Could you check a few things on this model? Use its own coordinates, in mm. Face numbers are marked on the shaded views. A direction names the side the tool comes from. Round coordinates to 2 decimals unless told otherwise and drop trailing zeros. Loops run counter-clockwise (first coordinate to the right, second up) from the corner with the lowest first, then second, coordinate; pieces in that order, holes last. Notation, with made-up numbers: (71.25, 72.5) -> (111.25, 72.5) arc R16 ccw to (111.25, 96.5) -> close; hole circle Ø1 at (51.5, 27). An arc over 180 degrees is marked (long way). Put each result on its own line as item: value. Start each with the question number.
1. I'm going to push flat-ended pins straight in: P1, Ø5, axis at x = -14, y = -21, coming from the +Z side; P2, Ø5, axis at x = 13, y = 12, coming from the -Z side; P3, Ø6, axis at x = 2, z = -4, coming from the -Y side. Where does each tip first touch, or does it pass through?
2. If we mould it in two halves opening along Z, with no side actions, what happens to the marked faces 4, 5 and 6? For each: pulls with the +Z half, pulls with the -Z half, needs draft (parallel to the pull), parting line crosses it, or undercut.
3. Which directions (+Z, -Z, +X, -X, +Y, -Y) give clear straight access to the entire face, cutting with the end or side of a thin tool? Please do the marked faces 1, 2 and 3.
4. Imagine slicing it at A-A, the plane y = 24.75. Please give me the cut outline in (x, z).
5. Imagine slicing it at B-B, the plane x = -24.75. Please give me the cut outline in (y, z).
6. Imagine slicing it at C-C, the plane z = 11. Please give me the cut outline in (x, y).
7. Imagine slicing it at D-D, the plane x = 0. Please give me the cut outline in (y, z).
8. I need wall thicknesses on line 1 (Y direction, x = -24.75, z = 28.5); line 2 (Z direction, x = -0.5, y = 3.5); line 3 (Y direction, x = -24, z = 8). Which ranges of each line are inside material? Lowest first, please. Write a range as [from, to].
```python
from build123d import *

# Parameters (mm, degrees)
BOSS_EXTRUDE1_DEPTH = 2.5
SKETCH3_W           = 45
SKETCH3_H           = 1.418134712
SKETCH3_W_2         = 44.463900584
SKETCH3_H_2         = 3.684459624
BOSS_EXTRUDE2_DEPTH = 31.5
SKETCH4_W           = 60.536099416
SKETCH4_H           = 60
BOSS_EXTRUDE3_DEPTH = 34
SKETCH5_R           = 21
BOSS_EXTRUDE4_DEPTH = 80
SKETCH6_R           = 4
BOSS_EXTRUDE5_DEPTH = 3
SKETCH7_R           = 15
BOSS_EXTRUDE6_DEPTH = 22
SKETCH13_R          = 2
CUT_EXTRUDE1_DEPTH  = 3
CUT_EXTRUDE2_START  = -3
SKETCH14_R          = 2
CUT_EXTRUDE2_DEPTH  = 3
SKETCH15_R          = 2.5
SKETCH15_W          = 52.231950292
SKETCH15_H          = 11.081865288
SKETCH15_W_2        = 52.768049708
SKETCH15_H_2        = 8.918134712
CUT_EXTRUDE3_DEPTH  = 128.185394164


with BuildPart() as part:
    # Sketch2 → Boss-Extrude1 (new body)
    with BuildSketch(Plane.XY):
        Polygon((-30.268049708, -30), (-30.268049708, 31.081865288), (-22.5, 31.081865288), (-22.5, 41.081865288), (21.963900584, 41.081865288), (21.963900584, 29.468648207), (29.731950292, 29.468648207), (29.731950292, -30.531351793), (22.5, -30.531351793), (22.5, -38.918134712), (-22.5, -38.918134712), (-22.5, -30), align=None)
    extrude(amount=BOSS_EXTRUDE1_DEPTH)

    # Sketch3 → Boss-Extrude2 (add)
    with BuildSketch(Plane.XY.offset(2.5)):
        with Locations((0, -38.209067356)):
            Rectangle(SKETCH3_W, SKETCH3_H)
        with Locations((-0.268049708, 39.239635476)):
            Rectangle(SKETCH3_W_2, SKETCH3_H_2)
    extrude(amount=BOSS_EXTRUDE2_DEPTH)

    # Sketch4 → Boss-Extrude3 (add)
    with BuildSketch(Plane.XY.offset(2.5)):
        Rectangle(SKETCH4_W, SKETCH4_H)
    extrude(amount=BOSS_EXTRUDE3_DEPTH)

    # Sketch5 → Boss-Extrude4 (add)
    with BuildSketch(Plane.XY.offset(36.5)):
        Circle(SKETCH5_R)
    extrude(amount=BOSS_EXTRUDE4_DEPTH)

    # Sketch6 → Boss-Extrude5 (add)
    with BuildSketch(Plane(origin=(0, 0, 0), x_dir=(-1, 0, 0), z_dir=(0, 0, -1))):
        with Locations((0, -10)):
            Circle(SKETCH6_R)
    extrude(amount=BOSS_EXTRUDE5_DEPTH)

    # Sketch7 → Boss-Extrude6 (add)
    with BuildSketch(Plane(origin=(0, 0, -3), x_dir=(-1, 0, 0), z_dir=(0, 0, -1))):
        with Locations((0, -10)):
            Circle(SKETCH7_R)
    extrude(amount=BOSS_EXTRUDE6_DEPTH)

    # Sketch13 → Cut-Extrude1 (cut)
    with BuildSketch(Plane(origin=(0, 41.081865288, 0), x_dir=(1, 0, 0), z_dir=(0, 1, 0))):
        with Locations(Location((-12.5, -14, 0), (0, 0, 270))):
            Circle(SKETCH13_R)
        with Locations(Location((12.5, -14, 0), (0, 0, 270))):
            Circle(SKETCH13_R)
        with Locations(Location((-12.5, -26, 0), (0, 0, 270))):
            Circle(SKETCH13_R)
        with Locations(Location((12.5, -26, 0), (0, 0, 270))):
            Circle(SKETCH13_R)
    extrude(amount=-CUT_EXTRUDE1_DEPTH, mode=Mode.SUBTRACT)

    # Sketch14 → Cut-Extrude2 (cut)
    with BuildSketch(Plane.XZ.offset(38.918134712).offset(CUT_EXTRUDE2_START)):
        with Locations(Location((12.5, 26, 0), (0, 0, 90))):
            Circle(SKETCH14_R)
        with Locations(Location((12.5, 14, 0), (0, 0, 90))):
            Circle(SKETCH14_R)
        with Locations(Location((-12.5, 14, 0), (0, 0, 90))):
            Circle(SKETCH14_R)
        with Locations(Location((-12.5, 26, 0), (0, 0, 90))):
            Circle(SKETCH14_R)
    extrude(amount=CUT_EXTRUDE2_DEPTH, mode=Mode.SUBTRACT)

    # Sketch15 → Cut-Extrude3 (cut, through all)
    with BuildSketch(Plane(origin=(0, 0, 0), x_dir=(-1, 0, 0), z_dir=(0, 0, -1))):
        with Locations((-24.75, 24.75)):
            Circle(SKETCH15_R)
        with Locations((24.75, 24.75)):
            Circle(SKETCH15_R)
        with Locations((24.75, -24.75)):
            Circle(SKETCH15_R)
        with Locations((-24.75, -24.75)):
            Circle(SKETCH15_R)
        with Locations((4.152074562, 35.540932644)):
            Rectangle(SKETCH15_W, SKETCH15_H)
        with Locations((3.884024854, -34.459067356)):
            Rectangle(SKETCH15_W_2, SKETCH15_H_2)
    extrude(amount=-CUT_EXTRUDE3_DEPTH, mode=Mode.SUBTRACT)


solid = part.part
```
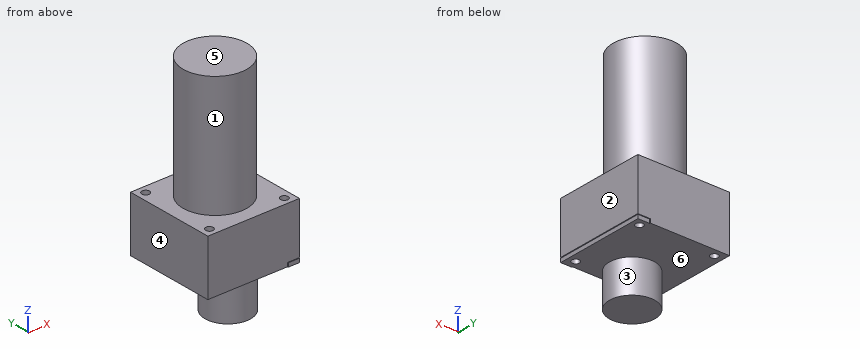
Entries:
1. P1: z = 36.5
1. P2: z = 0
1. P3: y = -25
2. face 4: needs draft
2. face 5: pulls with the +Z half
2. face 6: undercut
3. face 1: +Z
3. face 2: +Z, -Z, +X, +Y, -Y
3. face 3: -Z
4. outline: (-30.27, 0) -> (-27.25, 0) -> (-27.25, 36.5) -> (-30.27, 36.5) -> close; (-22.25, 0) -> (22.25, 0) -> (22.25, 36.5) -> (-22.25, 36.5) -> close; (27.25, 0) -> (29.73, 0) -> (29.73, 2.5) -> (30.27, 2.5) -> (30.27, 36.5) -> (27.25, 36.5) -> close
5. outline: (-30, 0) -> (-27.25, 0) -> (-27.25, 36.5) -> (-30, 36.5) -> close; (-22.25, 0) -> (22.25, 0) -> (22.25, 36.5) -> (-22.25, 36.5) -> close; (27.25, 0) -> (30, 0) -> (30, 36.5) -> (27.25, 36.5) -> close
6. outline: (-30.27, -30) -> (30.27, -30) -> (30.27, 30) -> (-30.27, 30) -> close; hole circle Ø5 at (-24.75, -24.75); hole circle Ø5 at (-24.75, 24.75); hole circle Ø5 at (24.75, -24.75); hole circle Ø5 at (24.75, 24.75)
7. outline: (-30, 0) -> (-14, 0) -> (-14, -3) -> (-25, -3) -> (-25, -25) -> (5, -25) -> (5, -3) -> (-6, -3) -> (-6, 0) -> (30, 0) -> (30, 36.5) -> (21, 36.5) -> (21, 116.5) -> (-21, 116.5) -> (-21, 36.5) -> (-30, 36.5) -> close
8. line 1: [-30, -27.25], [-22.25, 22.25], [27.25, 30]
8. line 2: [-25, -3], [0, 116.5]
8. line 3: [-30, -27.13], [-22.37, 22.37], [27.13, 30]
